Geometry check sheet. Reference: the model listing, model coordinates, mm. A direction names the side the tool comes from. Coordinates: 2 decimals unless noted, no trailing zeros. Write each loop counter-clockwise with the first axis right and the second up, starting at its lowest first coordinate (ties: lowest second). Pieces come first, ordered by that corner, then holes. Notation, with made-up numbers: (33.25, 85.25) -> (64.25, 85.25) arc R23 cw to (64.25, 119.25) -> close; hole circle Ø2 at (8, 37.25). An arc over 180 degrees is marked (long way). Use a Markdown table: item, result.
```python
from build123d import *

# Parameters (mm, degrees)
F1_DEPTH  = 56
F2_W      = 4
F2_H      = 38
F2_R      = 1.1
F2_R_2    = 12.5
F3_DEPTH  = 1
F4_W      = 21
F4_H      = 56
F4_R      = 1.1
F5_DEPTH  = 1
F6_W      = 20
F6_H      = 5
F7_DEPTH  = 1
F8_W      = 36
F8_H      = 38
F9_DEPTH  = 1
F11_R     = 1.1
F11_W     = 12
F11_H     = 32
F12_DEPTH = 1
F13_W     = 34.5
F13_H     = 1
F14_DEPTH = 10
F15_R     = 12.5
F15_W     = 15
F15_H     = 5
F16_DEPTH = 3.5
F18_DEPTH = 1
F19_R     = 1
F20_R     = 5


with BuildPart() as f1:
    # F0 (on Top) → F1 (new body)
    with BuildSketch(Plane.XY):
        Polygon((16.25, -20), (-16.25, -20), (-16.25, 20), (-17.25, 20), (-17.25, -21), (17.25, -21), (17.25, 20), (16.25, 20), align=None)
    extrude(amount=F1_DEPTH)

    # F2 (on face) → F3 (cut, through all)
    with BuildSketch(Plane(origin=(-17.25, 0, 0), x_dir=(0, -1, 0), z_dir=(-1, 0, 0))):
        Polygon((-20, 0), (20, 0), (20, 9), (-16, 9), (-20, 9), align=None)
        with Locations((-18, 28)):
            Rectangle(F2_W, F2_H)
        Polygon((-20, 56), (-20, 47), (-16, 47), (20, 47), (20, 56), align=None)
        with Locations((18, 43)):
            Circle(F2_R)
        with Locations((-12, 43)):
            Circle(F2_R)
        with Locations((-12, 13)):
            Circle(F2_R)
        with Locations((18, 13)):
            Circle(F2_R)
        with Locations((3, 28)):
            Circle(F2_R_2)
    extrude(amount=-F3_DEPTH, mode=Mode.SUBTRACT)

    # F4 (on face) → F5 (cut, through all)
    with BuildSketch(Plane.YZ.offset(17.25)):
        with Locations((9.5, 28)):
            Rectangle(F4_W, F4_H)
        with Locations((-6, 8)):
            Circle(F4_R)
        with Locations((-6, 48)):
            Circle(F4_R)
    extrude(amount=-F5_DEPTH, mode=Mode.SUBTRACT)

    # F6 (on face) → F7 (cut)
    with BuildSketch(Plane.YZ.offset(17.25)):
        with Locations((-11, 2.5)):
            Rectangle(F6_W, F6_H)
        with Locations((-11, 53.5)):
            Rectangle(F6_W, F6_H)
    extrude(amount=-F7_DEPTH, mode=Mode.SUBTRACT)

    # F8 (on face) → F9 (cut)
    with BuildSketch(Plane(origin=(-17.25, 0, 0), x_dir=(0, -1, 0), z_dir=(-1, 0, 0))):
        with Locations((2, 28)):
            Rectangle(F8_W, F8_H)
    extrude(amount=-F9_DEPTH, mode=Mode.SUBTRACT)

    # F10: F1 across plane


with BuildPart() as f1_1:
    add(f1.part)
    add(f1.part.mirror(Plane.YZ))

    # F11 (on face) → F12 (cut, through all)
    with BuildSketch(Plane(origin=(-17.25, 0, 0), x_dir=(0, -1, 0), z_dir=(-1, 0, 0))):
        with Locations((17, 43)):
            Circle(F11_R)
        with Locations((17, 13)):
            Circle(F11_R)
        with Locations((7, 28)):
            Rectangle(F11_W, F11_H)
    extrude(amount=-F12_DEPTH, mode=Mode.SUBTRACT)

    # F13 (on face) → F14 (join)
    with BuildSketch(Plane.XZ.offset(21)):
        with Locations((0, -0.5)):
            Rectangle(F13_W, F13_H)
        with Locations((0, 56.5)):
            Rectangle(F13_W, F13_H)
    extrude(amount=-F14_DEPTH)

    # F15 (on face) → F16 (cut)
    with BuildSketch(Plane.XZ.offset(21)):
        with Locations((0, 28)):
            Circle(F15_R)
        with Locations((0, 57)):
            Rectangle(F15_W, F15_H)
        with Locations((0, -1)):
            Rectangle(F15_W, F15_H)
    extrude(amount=-F16_DEPTH, mode=Mode.SUBTRACT)

    # F17 (on face) → F18 (cut, through all)
    with BuildSketch(Plane.YZ.offset(17.25)):
        with BuildLine():
            ThreePointArc((-13.5, 15.25), (-13.2071067812, 14.5428932188), (-12.5, 14.25))
            Line((-12.5, 14.25), (-9.5, 14.25))
            ThreePointArc((-9.5, 14.25), (-8.7928932188, 14.5428932188), (-8.5, 15.25))
            Line((-8.5, 15.25), (-8.5, 23.25))
            ThreePointArc((-8.5, 23.25), (-8.7928932188, 23.9571067812), (-9.5, 24.25))
            Line((-9.5, 24.25), (-12.5, 24.25))
            ThreePointArc((-12.5, 24.25), (-13.2071067812, 23.9571067812), (-13.5, 23.25))
            Line((-13.5, 23.25), (-13.5, 15.25))
        make_face()
        with BuildLine():
            ThreePointArc((-12.5, 41.75), (-13.2071067812, 41.4571067812), (-13.5, 40.75))
            Line((-13.5, 40.75), (-13.5, 32.75))
            ThreePointArc((-13.5, 32.75), (-13.2071067812, 32.0428932188), (-12.5, 31.75))
            Line((-12.5, 31.75), (-9.5, 31.75))
            ThreePointArc((-9.5, 31.75), (-8.7928932188, 32.0428932188), (-8.5, 32.75))
            Line((-8.5, 32.75), (-8.5, 40.75))
            ThreePointArc((-8.5, 40.75), (-8.7928932188, 41.4571067812), (-9.5, 41.75))
            Line((-9.5, 41.75), (-12.5, 41.75))
        make_face()
    extrude(amount=-F18_DEPTH, mode=Mode.SUBTRACT)

    # F19
    f19_edges = [f1_1.edges().sort_by_distance(p)[0] for p in [
        (-17.25, -11, 56.5),
        (17.25, -11, 56.5),
        (16.75, -1, 51),
        (16.75, -1, 5),
        (-16.75, -1, 5),
        (-16.75, -1, 12),
        (-16.75, -1, 51),
        (-16.75, -1, 44),
        (-17.25, -11, -0.5),
        (17.25, -11, -0.5),
        (7.5, -20.5, 1.5),
        (7.5, -17.5, -0.5),
        (-7.5, -20.5, 1.5),
        (-7.5, -17.5, -0.5),
        (7.5, -20.5, 54.5),
        (7.5, -17.5, 56.5),
        (-7.5, -17.5, 56.5),
        (-7.5, -20.5, 54.5),
    ]]
    fillet(f19_edges, radius=F19_R)

    # F20
    f20_edges = [f1_1.edges().sort_by_distance(p)[0] for p in [
        (-16.75, -13, 44),
        (-16.75, -13, 12),
    ]]
    fillet(f20_edges, radius=F20_R)


solid = f1_1.part
```
Item 1: Tool access check on faces 1 (the flat face through (-7.5, -19.8, 56.4)), 2 (the cylindrical face through (-16.76, -16.13, 12.33)), 3 (the flat face through (0, -16, 0)). Record the directions out of +Z, -Z, +X, -X, +Y, -Y that give a thin tool (end or side, any length) a straight path to the whole face; none if there is none.
Answer block:
| item | result |
|---|---|
| face 1 | +Z, -Y |
| face 2 | -X |
| face 3 | +X, -X, +Y |
Item 2: Thickness scan on L1, parallel to Z at x = -16.7, y = -17; L2, parallel to Z at x = 16.95, y = -6; L3, parallel to Z at x = -16.5, y = -6. Record the ranges inside material, lowest first. Write a range as [from, to].
Answer block:
| item | result |
|---|---|
| L1 | z = [-1, 0], [5, 11.9], [14.1, 41.9], [44.1, 51], [56, 57] |
| L2 | z = [5, 6.9], [9.1, 46.9], [49.1, 51] |
| L3 | z = [5, 6.9], [9.1, 12], [44, 46.9], [49.1, 51] |
Item 3: Depth check by flat-ended pin: P1, Ø6, axis at x = 12, z = 33.5, coming from the +Y side; P2, Ø0.8, axis at x = 2.5, y = -20.5, coming from the -Z side; P3, Ø1.1, axis at x = -16.5, y = -6, coming from the +Z side; P4, Ø15, axis at x = 0, z = 28, coming from the -Y side. Enter the tip coordinate at first touch or a pass-through.
Answer block:
| item | result |
|---|---|
| P1 | stops at y = -20 |
| P2 | stops at z = 1.5 |
| P3 | stops at z = 51 |
| P4 | passes through |
Item 4: Mould release check, pull along Z, two halves, no side actions. Record for faces 4 (the flat face through (0, -15, 57)), 5 (the flat face through (0, -20, 15)), 6 (the flat face through (7.5, -19.8, -0.4)): +Z half, -Z half, draft (parallel to the pull), parting line (faces both ways), or undercut.
Answer block:
| item | result |
|---|---|
| face 4 | +Z half |
| face 5 | undercut |
| face 6 | draft |
Item 5: Section check C-C on y = -6. Record the boundary of the cut face in (x, z), then the cut area to 3 significant figures.
Answer block:
| item | result |
|---|---|
| outline | (-17.25, 5) -> (-16.25, 5) -> (-16.25, 6.9) -> (-17.25, 6.9) -> close; (-17.25, 9.1) -> (-16.25, 9.1) -> (-16.25, 12) -> (-17.25, 12) -> close; (-17.25, 44) -> (-16.25, 44) -> (-16.25, 46.9) -> (-17.25, 46.9) -> close; (-17.25, 49.1) -> (-16.25, 49.1) -> (-16.25, 51) -> (-17.25, 51) -> close; (16.25, 5) -> (17.25, 5) -> (17.25, 6.9) -> (16.25, 6.9) -> close; (16.25, 9.1) -> (17.25, 9.1) -> (17.25, 46.9) -> (16.25, 46.9) -> close; (16.25, 49.1) -> (17.25, 49.1) -> (17.25, 51) -> (16.25, 51) -> close |
| area | 51.2 mm^2 |
Item 6: Section check D-D on x = -14.5. Record the boundary of the cut face in (y, z), then the cut area to 3 significant figures.
Answer block:
| item | result |
|---|---|
| outline | (-21, -1) -> (-11, -1) -> (-11, 0) -> (-20, 0) -> (-20, 56) -> (-11, 56) -> (-11, 57) -> (-21, 57) -> close |
| area | 76.0 mm^2 |
Item 7: Section check B-B on y = -14.75. Record the boundary of the cut face in (x, z), then the cut area to 3 significant figures.
Answer block:
| item | result |
|---|---|
| outline | (-17.25, -1) -> (17.25, -1) -> (17.25, 0) -> (-17.25, 0) -> close; (-17.25, 5) -> (-16.25, 5) -> (-16.25, 51) -> (-17.25, 51) -> close; (-17.25, 56) -> (17.25, 56) -> (17.25, 57) -> (-17.25, 57) -> close; (16.25, 5) -> (17.25, 5) -> (17.25, 51) -> (16.25, 51) -> close |
| area | 161 mm^2 |
Item 8: Section check A-A on z = 43. Record the boundary of the cut face in (x, y), then the cut area to 3 significant figures.
Answer block:
| item | result |
|---|---|
| outline | (-17.25, -21) -> (17.25, -21) -> (17.25, -1) -> (16.25, -1) -> (16.25, -20) -> (-16.25, -20) -> (-16.25, -18.1) -> (-17.25, -18.1) -> close; (-17.25, -15.9) -> (-16.25, -15.9) -> (-16.25, -11) -> (-17.25, -11) -> close |
| area | 60.3 mm^2 |
